Verification items for the finished model (mm, model axes). Coordinates: 2 decimals unless noted, no trailing zeros. Order: outer loops, then holes, each group sorted by start corner. A loop starts at its lowest first (then second) coordinate and runs counter-clockwise, first axis right, second up. Notation, with made-up numbers: (76.5, 43.25) -> (89.5, 43.25) arc R22 cw to (89.5, 57.25) -> close; hole circle Ø7 at (-29, 22). An arc over 180 degrees is marked (long way). Answer as CSV lines item,"result".
```python
from build123d import *

# Parameters (mm, degrees)
SKETCH_1_W          = 160
SKETCH_1_H          = 12
SKETCH_1_R          = 1.6
EXTRUDE_1_DEPTH     = 5
CHAMFER_1_SIZE      = 1
SKETCH_2_W          = 124.5
SKETCH_2_H          = 12
SKETCH_2_W_2        = 65
SKETCH_2_H_2        = 88
EXTRUDE_2_DEPTH     = 5
CHAMFER_2_SIZE      = 40
SKETCH_3_R          = 2.1
SKETCH_3_W          = 45
SKETCH_3_H          = 20
CUT_EXTRUDE_1_DEPTH = 226.124965297
CUT_EXTRUDE_2_DEPTH = 226.124965297
CUT_EXTRUDE_3_DEPTH = 226.124965297
FILLET_1_R          = 3
FILLET_2_R          = 1.5
SKETCH_6_R          = 1.55
CUT_EXTRUDE_4_DEPTH = 226.124965297
FILLET_3_R          = 10
SKETCH_7_R          = 1.6
CUT_EXTRUDE_5_DEPTH = 226.124965297


with BuildPart() as part:
    # 草图1 → 凸台-拉伸1 (new body)
    with BuildSketch(Plane.XY):
        Rectangle(SKETCH_1_W, SKETCH_1_H)
        with Locations((55, -3)):
            Circle(SKETCH_1_R, mode=Mode.SUBTRACT)
        with Locations((75, -3)):
            Circle(SKETCH_1_R, mode=Mode.SUBTRACT)
        with Locations((-75, -3)):
            Circle(SKETCH_1_R, mode=Mode.SUBTRACT)
        with Locations((-55, -3)):
            Circle(SKETCH_1_R, mode=Mode.SUBTRACT)
        with Locations(Location((-75, 3, 0), (0, 0, 180))):
            Circle(SKETCH_1_R, mode=Mode.SUBTRACT)
        with Locations(Location((-55, 3, 0), (0, 0, 180))):
            Circle(SKETCH_1_R, mode=Mode.SUBTRACT)
        with Locations(Location((55, 3, 0), (0, 0, 180))):
            Circle(SKETCH_1_R, mode=Mode.SUBTRACT)
        with Locations(Location((75, 3, 0), (0, 0, 180))):
            Circle(SKETCH_1_R, mode=Mode.SUBTRACT)
    extrude(amount=EXTRUDE_1_DEPTH)

    # 倒角1
    chamfer_1_edges = [part.edges().sort_by_distance(p)[0] for p in [
        (80, -6, 2.5),
        (80, 6, 2.5),
    ]]
    chamfer(chamfer_1_edges, length=CHAMFER_1_SIZE)


with BuildPart() as body_2:
    # 草图2 → 凸台-拉伸2 (new body)
    with BuildSketch(Plane(origin=(0, 0, 0), x_dir=(-1, 0, 0), z_dir=(0, 0, -1))):
        with Locations((142.25, 0)):
            Rectangle(SKETCH_2_W, SKETCH_2_H)
        with Locations((172, -50)):
            Rectangle(SKETCH_2_W_2, SKETCH_2_H_2)
    extrude(amount=-EXTRUDE_2_DEPTH)

    # Combine 1: union part
    add(part.part)

    # 倒角2
    chamfer_2_edges = [body_2.edges().sort_by_distance(p)[0] for p in [
        (-139.5, -6, 2.5),
    ]]
    chamfer(chamfer_2_edges, length=CHAMFER_2_SIZE)

    # 草图3 → 切除-拉伸1 (cut, through all)
    with BuildSketch(Plane(origin=(0, 0, 0), x_dir=(-1, 0, 0), z_dir=(0, 0, -1))):
        with Locations((144.5, -90)):
            Circle(SKETCH_3_R)
        with Locations((199.5, -90)):
            Circle(SKETCH_3_R)
        with Locations((144.5, 2)):
            Circle(SKETCH_3_R)
        with Locations((199.5, 2)):
            Circle(SKETCH_3_R)
        with Locations((172, -94)):
            Rectangle(SKETCH_3_W, SKETCH_3_H)
        with Locations((172, 6)):
            Rectangle(SKETCH_3_W, SKETCH_3_H)
    extrude(amount=-CUT_EXTRUDE_1_DEPTH, mode=Mode.SUBTRACT)

    # 草图4 → 切除-拉伸2 (cut, through all)
    with BuildSketch(Plane.XY.offset(5)):
        Polygon((-150.5, -17.780613901), (-166.174632994, -44), (-150.5, -70.219386099), align=None)
        Polygon((-186.50071995, -10), (-172, -34.255749735), (-157.49928005, -10), align=None)
        Polygon((-172, -53.744250265), (-186.50071995, -78), (-157.49928005, -78), align=None)
        Polygon((-193.5, -17.780613901), (-193.5, -70.219386099), (-177.825367006, -44), align=None)
    extrude(amount=-CUT_EXTRUDE_2_DEPTH, mode=Mode.SUBTRACT)

    # 草图5 → 切除-拉伸3 (cut, through all)
    with BuildSketch(Plane(origin=(0, 0, 0), x_dir=(-1, 0, 0), z_dir=(0, 0, -1))):
        Polygon((110.813708499, -6), (138.5, -33.686291501), (138.5, -6), align=None)
    extrude(amount=-CUT_EXTRUDE_3_DEPTH, mode=Mode.SUBTRACT)

    # 圆角1
    fillet_1_edges = [body_2.edges().sort_by_distance(p)[0] for p in [
        (-157.49928005, -10, 2.5),
        (-172, -34.255749735, 2.5),
        (-186.50071995, -10, 2.5),
        (-186.50071995, -78, 2.5),
        (-172, -53.744250265, 2.5),
        (-157.49928005, -78, 2.5),
        (-193.5, -17.780613901, 2.5),
        (-177.825367006, -44, 2.5),
        (-193.5, -70.219386099, 2.5),
        (-150.5, -17.780613901, 2.5),
        (-150.5, -70.219386099, 2.5),
        (-166.174632994, -44, 2.5),
        (-110.813708499, -6, 2.5),
        (-138.5, -6, 2.5),
        (-138.5, -33.686291501, 2.5),
    ]]
    fillet(fillet_1_edges, radius=FILLET_1_R)

    # 圆角2
    fillet_2_edges = [body_2.edges().sort_by_distance(p)[0] for p in [
        (-204.5, -94, 2.5),
        (-139.5, -94, 2.5),
        (80, -5, 2.5),
        (80, 5, 2.5),
        (79, 6, 2.5),
        (79, -6, 2.5),
        (-204.5, 6, 2.5),
        (-194.5, -94, 2.5),
        (-149.5, -94, 2.5),
        (-194.5, -84, 2.5),
        (-149.5, -84, 2.5),
        (-194.5, 6, 2.5),
        (-149.5, 6, 2.5),
        (-149.5, -4, 2.5),
        (-194.5, -4, 2.5),
    ]]
    fillet(fillet_2_edges, radius=FILLET_2_R)

    # 草图6 → 切除-拉伸4 (cut, through all)
    with BuildSketch(Plane(origin=(0, 0, 0), x_dir=(-1, 0, 0), z_dir=(0, 0, -1))):
        with Locations((109.5, 2)):
            Circle(SKETCH_6_R)
        with Locations((144.5, -38)):
            Circle(SKETCH_6_R)
        with Locations((29.5, 2)):
            Circle(SKETCH_6_R)
        with Locations((-35.5, 2)):
            Circle(SKETCH_6_R)
    extrude(amount=-CUT_EXTRUDE_4_DEPTH, mode=Mode.SUBTRACT)

    # 圆角3
    fillet_3_edges = [body_2.edges().sort_by_distance(p)[0] for p in [
        (-99.5, -6, 2.5),
        (-139.5, -46, 2.5),
    ]]
    fillet(fillet_3_edges, radius=FILLET_3_R)

    # 草图7 → 切除-拉伸5 (cut, through all)
    with BuildSketch(Plane.XY.offset(5)):
        with Locations((-192.5, -10)):
            Circle(SKETCH_7_R)
        with Locations((-198.5, -44)):
            Circle(SKETCH_7_R)
    extrude(amount=-CUT_EXTRUDE_5_DEPTH, mode=Mode.SUBTRACT)


solid = body_2.part
```
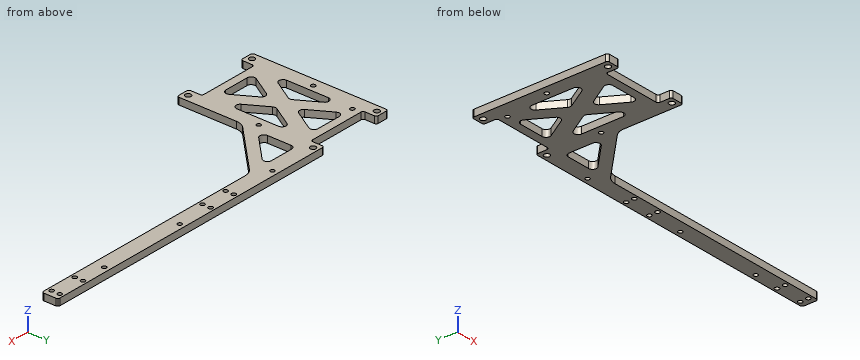
Item 1: Depth check by flat-ended pin: pin 1 Ø4 at (x, y) = (-144.5, 2) entering from +Z; pin 2 Ø3 at (x, z) = (-171.5, 4) entering from -Y; pin 3 Ø1.5 at (y, z) = (-78.5, 3.5) entering from +X; pin 4 Ø2.5 at (y, z) = (-17.5, 1.5) entering from +X. Enter the tip coordinate at first touch or a pass-through.
Answer list:
pin 1,"through"
pin 2,"y = -84"
pin 3,"x = -139.5"
pin 4,"x = -109.75"
Item 2: Section check A-A, the plane y = -66.5. Record the boundary of the cut face in (x, z).
Answer list:
outline,"(-204.5, 0) -> (-179.63, 0) -> (-179.63, 5) -> (-204.5, 5) -> close; (-164.37, 0) -> (-139.5, 0) -> (-139.5, 5) -> (-164.37, 5) -> close"
Item 3: Thickness scan on line 1 (Y direction, x = -55, z = 2.25); line 2 (Y direction, x = -153, z = 3.45); line 3 (Y direction, x = -163.5, z = 1.8). Record the ranges inside material, lowest first.
Answer list:
line 1,"-6 to -4.6, -1.4 to 1.4, 4.6 to 6"
line 2,"-84 to -62.31, -25.69 to -4"
line 3,"-84 to -78, -67.96 to -48.47, -39.53 to -20.04, -10 to -4"
Item 4: Section check B-B, the plane x = -125. Record the boundary of the cut face in (y, z).
Answer list:
outline,"(-31.5, 0) -> (-20.19, 0) -> (-20.19, 5) -> (-31.5, 5) -> close; (-6, 0) -> (6, 0) -> (6, 5) -> (-6, 5) -> close"
Item 5: Section check C-C, the plane z = 2.8. Count the separate pieces of the cut face and the enclosed holes in it, plus the area to 3 significant figures.
Answer list:
separate pieces,"1"
enclosed holes,"23"
area,"7,110 mm2"
